Autodesk Inventor part; units mm, degrees
ref_plane "YZ Plane" through (0, 0, 0) normal (1, 0, 0) x (0, 1, 0)
ref_plane "XZ Plane" through (0, 0, 0) normal (0, 1, 0) x (-1, 0, 0)
ref_plane "XY Plane" through (0, 0, 0) normal (0, 0, 1) x (1, 0, 0)
sketch "Sketch1" plane through (0, 0, 0) normal (0, 0, 1) x (1, 0, 0)
  line L0 (0, 0) -> (400, 0)
  line L1 (400, 0) -> (400, 300)
  line L2 (400, 300) -> (0, 300)
  line L3 (0, 300) -> (0, 0)
  line L4 (0, 0) -> (-10, 0)
  line L5 (-10, 0) -> (410, 0)
  line L6 (410, 0) -> (410, 310)
  line L7 (410, 310) -> (-10, 310)
  line L8 (-10, 310) -> (-10, 0)
  dimension "d0" = 400
  dimension "d1" = 300
  dimension "d4" = 10
extrude "Extrusion1" add sketch "Sketch1" against normal blind 400
extrude "Extrusion2" cut sketch "Sketch1" against normal blind 400 contours L3 L2 L1 L0
properties part number "Tunnel"
The listing builds one solid part. Answer for the finished solid, in the listing's coordinates (mm). A direction names the side the tool comes from. Coordinates: 2 decimals unless noted, no trailing zeros. Order: outer loops, then holes, each group sorted by start corner. A loop starts at its lowest first (then second) coordinate and runs counter-clockwise, first axis right, second up.
Q1. Which of the six approach directions +Z, -Z, +X, -X, +Y, -Y give full straight-line access (tool end or side, diameter ignored) to faces 1 (the face through (400, 148, -197)), 2 (the face through (-5, 0, -197))?
Q2. A cutting plane is placed at B-B, the plane z = -375. Write down the section's boundary in (x, y), and give its area (3 significant figures).
Q3. For a pull along X with two mould halves and no side action, classify faces 3 (the face through (405, 0, -197)), 4 (the face through (-10, 157, -197)), 5 (the face through (0, 152, -197)), 6 (the face through (203, 300, -197)) as pulls with the +X half, pulls with the -X half, needs draft (parallel to the pull), parting line crosses it, or undercut.
Q4. A cutting plane is placed at A-A, the plane y = 261. Write down the section's boundary in (x, z), and give its area (3 significant figures).
Q5. Given P1, Ø8, axis at x = 232, z = -294, coming from the -Y side, flat-ended and moving along its own axis, determine where the tip first touches the part or whether it passes through.
Q6. A cutting plane is placed at C-C, the plane x = 237. Write down the section's boundary in (y, z).
Q7. Consider line 1 (X direction, y = 75, z = -118); line 2 (Y direction, x = 108.5, z = -97.5). Determine where each line is inside the solid, lowest interval first.
Answers follow:
1. face 1: +Z, -Z, -Y
1. face 2: +Z, -Z, +X, -X, -Y
2. outline: (-10, 0) - (0, 0) - (0, 300) - (400, 300) - (400, 0) - (410, 0) - (410, 310) - (-10, 310) - close
2. area: 10,200 mm2
3. face 3: needs draft
3. face 4: pulls with the -X half
3. face 5: undercut
3. face 6: undercut
4. outline: (-10, -400) - (0, -400) - (0, 0) - (-10, 0) - close; (400, -400) - (410, -400) - (410, 0) - (400, 0) - close
4. area: 8,000 mm2
5. P1: stops at y = 300
6. outline: (300, -400) - (310, -400) - (310, 0) - (300, 0) - close
7. line 1: x = -10 to 0, 400 to 410
7. line 2: y = 300 to 310
